from build123d import *

# Parameters (mm, degrees)
BOSS_EXTRUDE1_DEPTH = 3
CUT_EXTRUDE2_REACH  = 5
SKETCH2_R           = 2


with BuildPart() as part:
    # Sketch1 → Boss-Extrude1 (new body)
    with BuildSketch(Plane(origin=(110.5, 0, 0), x_dir=(0, 0, -1), z_dir=(1, 0, 0))):
        with BuildLine():
            Line((122.5, 328.5), (122.5, -10))
            Line((122.5, -10), (-227.5, -10))
            ThreePointArc((-227.5, -10), (-231.293387843, -8.070194473), (-231.967157887, -3.867817213))
            Line((-231.967157887, -3.867817213), (-125.468557887, 326.745775479))
            ThreePointArc((-125.468557887, 326.745775479), (-123.764798126, 329.10018419), (-121.0014, 330))
            Line((-121.0014, 330), (121, 330))
            ThreePointArc((121, 330), (122.060660172, 329.560660172), (122.5, 328.5))
        make_face()
    extrude(amount=-BOSS_EXTRUDE1_DEPTH)

    # Sketch2 → Cut-Extrude2 (cut, up to next)
    with BuildSketch(Plane(origin=(110.5, 0, 0), x_dir=(0, 0, -1), z_dir=(1, 0, 0)), mode=Mode.PRIVATE) as cut_extrude2_sk1:
        with Locations((111.5014, 297.910969137)):
            Circle(SKETCH2_R)
    cut_extrude2_tool1 = extrude(cut_extrude2_sk1.sketch, amount=-CUT_EXTRUDE2_REACH, mode=Mode.PRIVATE) & part.part
    add(cut_extrude2_tool1.solids().sort_by_distance((110.5, 297.910969, -111.5014))[0], mode=Mode.SUBTRACT)
    # Sketch2 → Cut-Extrude2 (cut, up to next)
    with BuildSketch(Plane(origin=(110.5, 0, 0), x_dir=(0, 0, -1), z_dir=(1, 0, 0)), mode=Mode.PRIVATE) as cut_extrude2_sk2:
        with Locations((90.410969137, 0.9986)):
            Circle(SKETCH2_R)
    cut_extrude2_tool2 = extrude(cut_extrude2_sk2.sketch, amount=-CUT_EXTRUDE2_REACH, mode=Mode.PRIVATE) & part.part
    add(cut_extrude2_tool2.solids().sort_by_distance((110.5, 0.9986, -90.410969))[0], mode=Mode.SUBTRACT)
    # Sketch2 → Cut-Extrude2 (cut, up to next)
    with BuildSketch(Plane(origin=(110.5, 0, 0), x_dir=(0, 0, -1), z_dir=(1, 0, 0)), mode=Mode.PRIVATE) as cut_extrude2_sk3:
        with Locations((-209.589030863, 0.9986)):
            Circle(SKETCH2_R)
    cut_extrude2_tool3 = extrude(cut_extrude2_sk3.sketch, amount=-CUT_EXTRUDE2_REACH, mode=Mode.PRIVATE) & part.part
    add(cut_extrude2_tool3.solids().sort_by_distance((110.5, 0.9986, 209.589031))[0], mode=Mode.SUBTRACT)
    # Sketch2 → Cut-Extrude2 (cut, up to next)
    with BuildSketch(Plane(origin=(110.5, 0, 0), x_dir=(0, 0, -1), z_dir=(1, 0, 0)), mode=Mode.PRIVATE) as cut_extrude2_sk4:
        with Locations((-113.4986, 297.910969137)):
            Circle(SKETCH2_R)
    cut_extrude2_tool4 = extrude(cut_extrude2_sk4.sketch, amount=-CUT_EXTRUDE2_REACH, mode=Mode.PRIVATE) & part.part
    add(cut_extrude2_tool4.solids().sort_by_distance((110.5, 297.910969, 113.4986))[0], mode=Mode.SUBTRACT)


solid = part.part
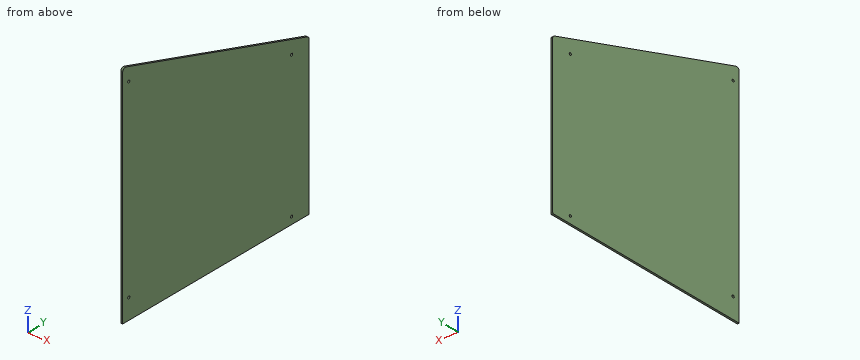
Input: part model. Units: mm. Frame: model coordinates. Give positions to 0.01 mm unless a question says otherwise; leave off trailing zeros. Order: outer loops, then holes, each group sorted by start corner. A loop starts at its lowest first (then second) coordinate and runs counter-clockwise, first axis right, second up.
Q1. Contact query for a flat-ended pin moving along its axis: pin 1 Ø1 at (x, y) = (109, 208) entering from +Z. Output: stop coordinate, or through.
Checked values:
pin 1: stops at z = 163.88
Q2. Section B-B on y = 19. Output: boundary loops of the cut face in (x, z), and give its area (3 significant figures).
Checked values:
outline: (107.5, -122.5) - (110.5, -122.5) - (110.5, 224.6) - (107.5, 224.6) - close
area: 1,040 mm2
Q3. Section C-C on z = 172. Output: boundary loops of the cut face in (x, y), and give its area (3 significant figures).
Checked values:
outline: (107.5, -10) - (110.5, -10) - (110.5, 182.29) - (107.5, 182.29) - close
area: 577 mm2
Q4. Section A-A on x = 108.6. Output: boundary loops of the cut face in (y, z).
Checked values:
outline: (-10, -122.5) - (328.5, -122.5) arc R1.5 ccw to (330, -121) - (330, 121) arc R4.69 ccw to (326.75, 125.47) - (-3.87, 231.97) arc R4.69 ccw to (-10, 227.5) - close; hole circle Ø4 at (1, -90.41); hole circle Ø4 at (1, 209.59); hole circle Ø4 at (297.91, -111.5); hole circle Ø4 at (297.91, 113.5)
Q5. Ray query, probe 1 along Z at (x, y) = (107.7, 316); probe 2 along Z at (x, y) = (108.8, 189). Return the intervals inside material, ascending.
Checked values:
probe 1: z = -122.5 to 128.93
probe 2: z = -122.5 to 169.84
